For this review, use the dimensioned drawing (mm, ordinates from the lowest corner) and the shaded views. Coordinates: 2 decimals unless noted, no trailing zeros. Loops run counter-clockwise (first coordinate to the right, second up) from the corner with the lowest first, then second, coordinate; pieces in that order, holes last. Notation, with made-up numbers: (76.5, 73) - (127.5, 73) arc R7 ccw to (127.5, 84) - close; hole circle Ø4 at (61, -32.75). An arc over 180 degrees is marked (long way). Answer in a Markdown table with one row per item. Add a question column.
(1) We need section A-A, the plane y = 29. Write out the cut boundary in (x, z) (1 decimal), plus the area to 3 significant figures.
(2) We need section B-B, the plane x = 59. Write out the cut boundary in (y, z) (1 decimal).
(3) Clearance check with flat-ended pins moving along their axes: pin 1 (5 mm diameter, centred on x = 71, z = 15.5, fed in from +Y); pin 2 (6 mm diameter, centred on x = 33.5, z = 11.5, fed in from +Y); pin 3 (8 mm diameter, centred on y = 12.5, z = 13.5, fed in from +X). State where each tip first meets the part, or that it passes through.
(4) To check wall thickness, follow L1, parallel to Y at x = 39, z = 17.5 (1 decimal); L2, parallel to X at y = 48, z = 18 (1 decimal); L3, parallel to Y at x = 32, z = 23.5 (1 decimal). State the ranges of each line that lie inside material, in increasing order. Write a range as [from, to].
(5) We need section D-D, the plane x = 84.5. Write out the cut boundary in (y, z).
(6) The part is to be moulded in two halves that separate along X. For the marked faces 1, 2, 3 and 4, say which applies: released by +X, released by -X, zero draft, split by the parting line, or undercut.
(7) We need section C-C, the plane z = 10.75. Write out the cut boundary in (x, y) (1 decimal), plus the area to 3 significant figures.
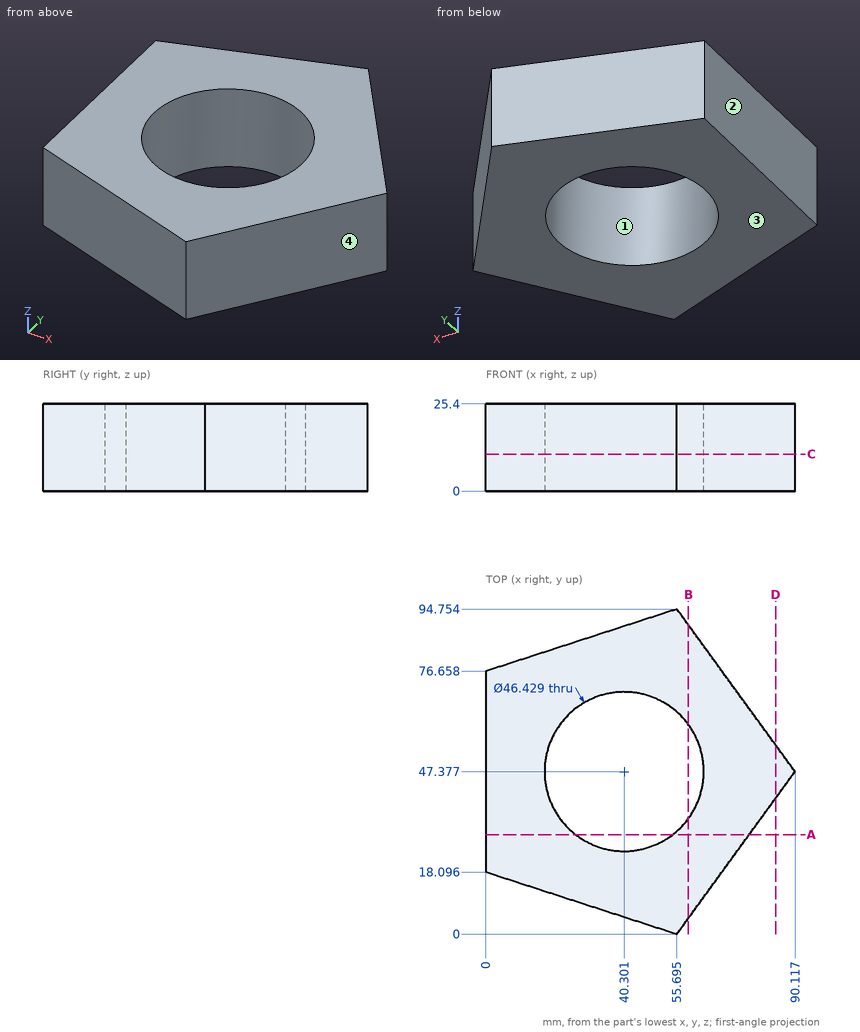
Responses:
| question | item | result |
|---|---|---|
| 1 | outline | (0, 0) - (26.1, 0) - (26.1, 25.4) - (0, 25.4) - close; (54.5, 0) - (76.8, 0) - (76.8, 25.4) - (54.5, 25.4) - close |
| 1 | area | 1,230 mm2 |
| 2 | outline | (4.5, 0) - (33.6, 0) - (33.6, 25.4) - (4.5, 25.4) - close; (61.1, 0) - (90.2, 0) - (90.2, 25.4) - (61.1, 25.4) - close |
| 3 | pin 1 | stops at y = 77.13 |
| 3 | pin 2 | stops at y = 88.52 |
| 3 | pin 3 | stops at x = 67.68 |
| 4 | L1 | y = [5.4, 24.2], [70.6, 89.3] |
| 4 | L2 | x = [0, 17.1], [63.5, 89.7] |
| 4 | L3 | y = [7.7, 25.7], [69.1, 87.1] |
| 5 | outline | (39.65, 0) - (55.11, 0) - (55.11, 25.4) - (39.65, 25.4) - close |
| 6 | face 1 | undercut |
| 6 | face 2 | released by -X |
| 6 | face 3 | zero draft |
| 6 | face 4 | released by +X |
| 7 | outline | (0, 18.1) - (55.7, 0) - (90.1, 47.4) - (55.7, 94.8) - (0, 76.7) - close; hole circle Ø46.4 at (40.3, 47.4) |
| 7 | area | 4,210 mm2 |
